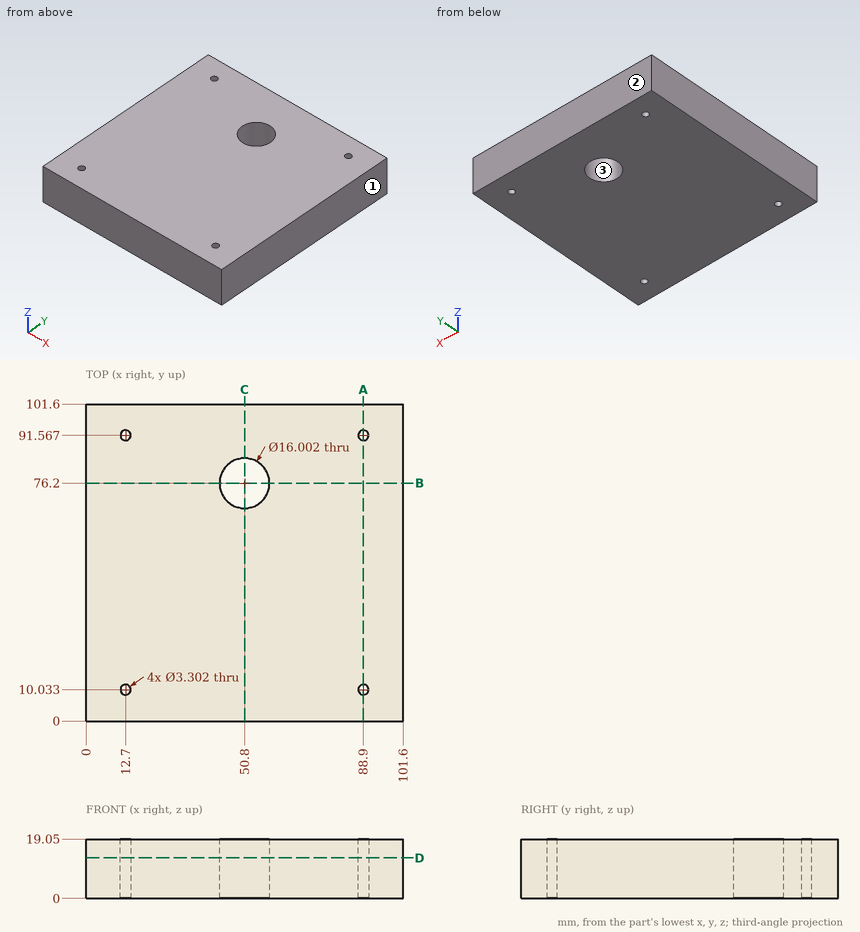
Check sheet for the drawn part. Datum: minimum x, y, z corner. Units: mm. Give positions to 0.01 mm unless a question says otherwise; leave off trailing zeros. Order: outer loops, then holes, each group sorted by start corner. A loop starts at its lowest first (then second) coordinate and runs counter-clockwise, first axis right, second up. Notation, with made-up numbers: (81.5, 54.25) -> (106.5, 54.25) arc R27 ccw to (106.5, 73.25) -> close; hole circle Ø5 at (-6, 41). An arc over 180 degrees is marked (long way). Use a Markdown table: item, result.
1) Section check C-C, the plane x = 50.8. Record the boundary of the cut face in (y, z), then the cut area to 3 significant figures.
Results:
| item | result |
|---|---|
| outline | (0, 0) -> (68.2, 0) -> (68.2, 19.05) -> (0, 19.05) -> close; (84.2, 0) -> (101.6, 0) -> (101.6, 19.05) -> (84.2, 19.05) -> close |
| area | 1,630 mm² |
2) Material ranges on probe 1 along Y at (x, z) = (12.7, 14); probe 2 along Y at (x, z) = (52, 10.25); probe 3 along X at (y, z) = (80.5, 15), recorded low to high.
Results:
| item | result |
|---|---|
| probe 1 | 0 to 8.38, 11.68 to 89.92, 93.22 to 101.6 |
| probe 2 | 0 to 68.29, 84.11 to 101.6 |
| probe 3 | 0 to 44.05, 57.55 to 101.6 |
3) Section check B-B, the plane y = 76.2. Record the boundary of the cut face in (x, z), then the cut area to 3 significant figures.
Results:
| item | result |
|---|---|
| outline | (0, 0) -> (42.8, 0) -> (42.8, 19.05) -> (0, 19.05) -> close; (58.8, 0) -> (101.6, 0) -> (101.6, 19.05) -> (58.8, 19.05) -> close |
| area | 1,630 mm² |
4) Section check A-A, the plane x = 88.9. Record the boundary of the cut face in (y, z), then the cut area to 3 significant figures.
Results:
| item | result |
|---|---|
| outline | (0, 0) -> (8.38, 0) -> (8.38, 19.05) -> (0, 19.05) -> close; (11.68, 0) -> (89.92, 0) -> (89.92, 19.05) -> (11.68, 19.05) -> close; (93.22, 0) -> (101.6, 0) -> (101.6, 19.05) -> (93.22, 19.05) -> close |
| area | 1,810 mm² |
5) Mould release check, pull along X, two halves, no side actions. Record for the marked faces 1, 2 and 3: pulls with the +X half, pulls with the -X half, needs draft (parallel to the pull), parting line crosses it, or undercut.
Results:
| item | result |
|---|---|
| face 1 | pulls with the +X half |
| face 2 | needs draft |
| face 3 | undercut |
6) Depth check by flat-ended pin: pin 1 Ø5.5 at (x, y) = (12.7, 91.567) entering from +Z; pin 2 Ø2.5 at (x, y) = (88.9, 10.033) entering from +Z. Enter the tip coordinate at first touch or a pass-through.
Results:
| item | result |
|---|---|
| pin 1 | z = 19.05 |
| pin 2 | through |
7) Section check D-D, the plane z = 13. Record the boundary of the cut face in (x, y), then the cut area to 3 significant figures.
Results:
| item | result |
|---|---|
| outline | (0, 0) -> (101.6, 0) -> (101.6, 101.6) -> (0, 101.6) -> close; hole circle Ø3.3 at (12.7, 10.03); hole circle Ø3.3 at (12.7, 91.57); hole circle Ø16 at (50.8, 76.2); hole circle Ø3.3 at (88.9, 10.03); hole circle Ø3.3 at (88.9, 91.57) |
| area | 10,100 mm² |
